from build123d import *

# Parameters (mm, degrees)
SKETCH1_R          = 3.25
SKETCH1_R_2        = 2.1
BASE_EXTRUDE_DEPTH = 1.2
SLIT_BEND_DEPTH    = 5.750263151


with BuildPart() as part:
    # Sketch1 → Base-Extrude (new body)
    with BuildSketch(Plane(origin=(0, 0, 0), x_dir=(0, 0, -1), z_dir=(1, 0, 0))):
        Circle(SKETCH1_R)
        Circle(SKETCH1_R_2, mode=Mode.SUBTRACT)
    extrude(amount=BASE_EXTRUDE_DEPTH)

    # Sketch2 → Slit-bend (cut, through all)
    with BuildSketch(Plane(origin=(0, 0, 0), x_dir=(0, 0, -1), z_dir=(1, 0, 0))):
        with BuildLine():
            Line((-0.125, -2.096276461), (-0.125, -3.247595264))
            ThreePointArc((-0.125, -3.247595264), (0, -3.25), (0.125, -3.247595264))
            Line((0.125, -3.247595264), (0.125, -2.096276461))
            ThreePointArc((0.125, -2.096276461), (0, -2.1), (-0.125, -2.096276461))
        make_face()
    extrude(amount=SLIT_BEND_DEPTH, mode=Mode.SUBTRACT)


solid = part.part
CAD build for the part. Positions are in the model's coordinates, mm. A direction names the side the tool comes from. Give positions to 0.01 mm unless a question says otherwise; leave off trailing zeros. Write each loop counter-clockwise with the first axis right and the second up, starting at its lowest first coordinate (ties: lowest second). Pieces come first, ordered by that corner, then holes. Notation, with made-up numbers: (89, 33.5) - (108, 33.5) arc R13 ccw to (108, 44.5) - close; hole circle Ø1 at (-37, 64.5). An arc over 180 degrees is marked (long way). Answer as CSV lines item,"result".
Q1. Band-saw the part on C-C (z = 0). Give the cut face in (x, y), and give its area (3 significant figures).
Result set:
outline,"(0, 2.1) - (1.2, 2.1) - (1.2, 3.25) - (0, 3.25) - close"
area,"1.38 mm²"
Q2. Band-saw the part on D-D (x = 0.95). Give the cut face in (y, z) (3 decimals), and give its area (3 significant figures).
Result set:
outline,"(-3.248, -0.125) arc R3.25 ccw (long way) to (-3.248, 0.125) - (-2.096, 0.125) arc R2.1 cw (long way) to (-2.096, -0.125) - close"
area,"19.0 mm²"
Q3. Pull direction Z, two halves, no side cores. Call faces 1 (the face through (0, 0.77, -2.12)), 2 (the face through (1, -3, 0.125)): released by +Z, released by -Z, zero draft, split by the parting line, or undercut.
Result set:
face 1,"zero draft"
face 2,"undercut"
Q4. Drill centre lines: line 1 (Z direction, x = 0.55, y = 0); line 2 (Y direction, x = 0.7, z = -0.25); line 3 (Y direction, x = 0.4, z = 0). Where is each one in solid material? Low to high. Write a range as from..to.
Result set:
line 1,"-3.25..-2.1, 2.1..3.25"
line 2,"-3.24..-2.09, 2.09..3.24"
line 3,"2.1..3.25"
Q5. 3-axis set-ups, long thin cutter, end or side, ignore diameter. For faces 3 (the face through (1, -3, -0.125)), 4 (the face through (1.2, 0.77, -2.12)): which of +Z, -Z, +X, -X, +Y, -Y reach the whole face in a straight line?
Result set:
face 3,"+X, -X, -Y"
face 4,"+Z, -Z, +X, +Y, -Y"
Q6. Flat gauge pin, fed straight in: pin 1 Ø0.6 at (x, y) = (0.5, -2.5) entering from +Z. Where does the tip first touch, or does it go through?
Result set:
pin 1,"z = 2.39"
Q7. Band-saw the part on A-A (z = -0.75). Give the cut face in (x, y), and give its area (3 significant figures).
Result set:
outline,"(0, -3.16) - (1.2, -3.16) - (1.2, -1.96) - (0, -1.96) - close; (0, 1.96) - (1.2, 1.96) - (1.2, 3.16) - (0, 3.16) - close"
area,"2.88 mm²"
Q8. Band-saw the part on B-B (y = 2). Give the cut face in (x, z).
Result set:
outline,"(0, -2.56) - (1.2, -2.56) - (1.2, -0.64) - (0, -0.64) - close; (0, 0.64) - (1.2, 0.64) - (1.2, 2.56) - (0, 2.56) - close"
